CAD build for the part. Positions are in the model's coordinates, mm. A direction names the side the tool comes from. Round coordinates to 2 decimals unless told otherwise and drop trailing zeros. Loops run counter-clockwise (first coordinate to the right, second up) from the corner with the lowest first, then second, coordinate; pieces in that order, holes last.
from build123d import *

# Parameters (mm, degrees)
SKETCH_1_R      = 6
EXTRUDE_1_DEPTH = 44
EXTRUDE_START   = 16
SKETCH_2_R      = 8.5
EXTRUDE_2_DEPTH = 6


with BuildPart() as part:
    # 草图1 → 凸台-拉伸1 (new body)
    with BuildSketch(Plane.XY):
        Circle(SKETCH_1_R)
    extrude(amount=EXTRUDE_1_DEPTH)

    # 草图2 → 凸台-拉伸2 (add)
    with BuildSketch(Plane.XY.offset(EXTRUDE_START)):
        Circle(SKETCH_2_R)
    extrude(amount=EXTRUDE_2_DEPTH)


solid = part.part
Item 1: 3-axis set-ups, long thin cutter, end or side, ignore diameter. For faces 1 (the flat face through (0, 0, 44)), 2 (the flat face through (2, 6, 16)), 3 (the cylindrical face through (-6, 0, 33)): which of +Z, -Z, +X, -X, +Y, -Y reach the whole face in a straight line?
Verdict:
face 1: +Z, +X, -X, +Y, -Y
face 2: -Z
face 3: +Z
Item 2: Cut at A-A (y = 0). List the corners of the cut face in (x, z).
Verdict:
outline: (-8.5, 16) - (-6, 16) - (-6, 0) - (6, 0) - (6, 16) - (8.5, 16) - (8.5, 22) - (6, 22) - (6, 44) - (-6, 44) - (-6, 22) - (-8.5, 22) - close
Item 3: Flat gauge pins, fed straight in: P1, Ø5, axis at y = 3.5, z = 6, coming from the +X side; P2, Ø10, axis at y = -5.5, z = 37.5, coming from the -X side; P3, Ø5, axis at x = 5, z = 11.5, coming from the +Y side. Where does each tip first touch, or does it go through?
Verdict:
P1: stops at x = 5.92
P2: stops at x = -5.98
P3: stops at y = 5.45
Item 4: Cut at C-C (z = 7). List the corners of the cut face in (x, y).
Verdict:
outline: circle Ø12 at (0, 0)
Item 5: Wall check: L1, parallel to X at y = 0.25, z = 38.5; L2, parallel to Z at x = 1.5, y = 6; L3, parallel to Y at x = -2.75, z = 8. Give the ranges that are in metal, low to high.
Verdict:
L1: x = -5.99 to 5.99
L2: z = 16 to 22
L3: y = -5.33 to 5.33
Item 6: Cut at D-D (y = 6.5). List the corners of the cut face in (x, z), plus the area to 3 significant figures.
Verdict:
outline: (-5.48, 16) - (5.48, 16) - (5.48, 22) - (-5.48, 22) - close
area: 65.7 mm2
